The model under review builds one solid part; all positions refer to its coordinate system, in mm. Face numbers are marked on the shaded views. A direction names the side the tool comes from. Give positions to 0.01 mm unless a question says otherwise; leave off trailing zeros. Return JSON: item names as keys, results as strings. Group by question number.
from build123d import *

# Parameters (mm, degrees)
SKETCH1_W           = 30
SKETCH1_H           = 12
BOSS_EXTRUDE1_DEPTH = 5
CUT_EXTRUDE1_DEPTH  = 34.823069051
LPATTERN1_COUNT     = 10
LPATTERN1_PITCH     = 3.141592654
TAP1_D              = 2.459
TAP1_DEPTH          = 6
TAP1_TIP            = 0.738758131
TAP3_D              = 2.459
TAP3_DEPTH          = 6
TAP3_TIP            = 0.738758131


with BuildPart() as part:
    # Sketch1 → Boss-Extrude1 (new, symmetric)
    with BuildSketch(Plane.XY):
        with Locations((15, 6)):
            Rectangle(SKETCH1_W, SKETCH1_H)
    extrude(amount=BOSS_EXTRUDE1_DEPTH, both=True)

    # Sketch2 → Cut-Extrude1 (cut, through all)
    with BuildSketch(Plane.XY.offset(5)):
        with BuildLine():
            Line((-1.149368398, 12), (1.149368398, 12))
            Line((1.149368398, 12), (0.426229404, 10.013191943))
            ThreePointArc((0.426229404, 10.013191943), (0.27978293, 9.822339182), (0.050352355, 9.75))
            Line((0.050352355, 9.75), (-0.050352355, 9.75))
            ThreePointArc((-0.050352355, 9.75), (-0.27978293, 9.822339182), (-0.426229404, 10.013191943))
            Line((-0.426229404, 10.013191943), (-1.149368398, 12))
        make_face()
    cut_extrude1 = extrude(amount=-CUT_EXTRUDE1_DEPTH, mode=Mode.SUBTRACT)

    # LPattern1: Cut-Extrude1 ×10
    with Locations(*[(i * LPATTERN1_PITCH, 0, 0) for i in range(1, LPATTERN1_COUNT)]):
        add(cut_extrude1, mode=Mode.SUBTRACT)

    # Tap1
    with Locations(Plane(origin=(-45.41658703, 4.630780207, 5), x_dir=(-1, 0, 0), z_dir=(0, 0, 1))):
        with Locations((-55.41658703, -0.869219793)):
            Hole(TAP1_D / 2, depth=TAP1_DEPTH)
            with Locations((0, 0, -(TAP1_DEPTH + TAP1_TIP / 2))):  # 118° drill point
                Cone(0, TAP1_D / 2, TAP1_TIP, mode=Mode.SUBTRACT)

    # Tap3
    with Locations(Plane(origin=(-24.792169361, 5.708678804, 5), x_dir=(-1, 0, 0), z_dir=(0, 0, 1))):
        with Locations((-49.792169361, 0.208678804)):
            Hole(TAP3_D / 2, depth=TAP3_DEPTH)
            with Locations((0, 0, -(TAP3_DEPTH + TAP3_TIP / 2))):  # 118° drill point
                Cone(0, TAP3_D / 2, TAP3_TIP, mode=Mode.SUBTRACT)


solid = part.part
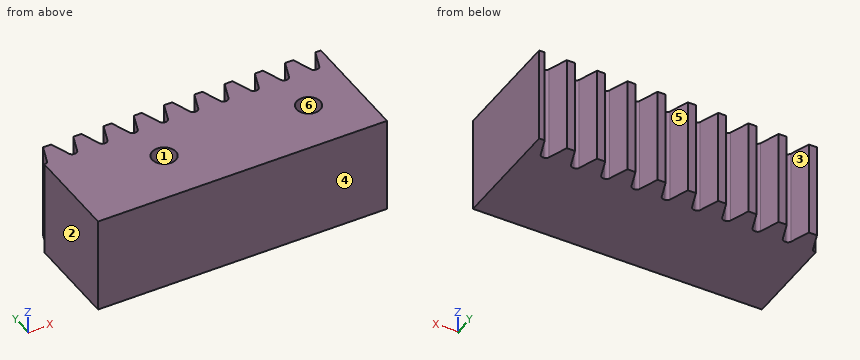
Item 1: Take a section at A-A (z = -0.25). State how many separate pieces and enclosed holes the cut face has, then the cut area to 3 significant figures.
Item 2: Mouldability with a two-part tool opening along Y and no side actions: class the marked faces 4, 5 and 6 as +Y half, -Y half, draft (parallel to the pull), parting line (faces both ways), or undercut.
Item 3: For L1, parallel to X at y = 5.5, z = 3.2; L2, parallel to Y at x = 12.25, z = -4.5; L3, parallel to Y at x = 25, z = 2.25, list the stretches that pass through material, from the lowest coordinate up. Write a range as from..to.
Item 4: Tool access review of the marked faces 1, 2 and 3: name each direction out of +Z, -Z, +X, -X, +Y, -Y from which nothing blocks a thin tool from reaching the whole face with its end or side.
Item 5: For P1, Ø2, axis at x = 25, y = 5.5, coming from the +Z side, flat-tipped, find the tip position at first contact; note if it passes through.
Check sheet entries:
{
 "1": {"separate pieces": "1", "enclosed holes": "2", "area": "319 mm^2"},
 "2": {"face 4": "-Y half", "face 5": "+Y half", "face 6": "undercut"},
 "3": {"L1": "x = 0..8.77, 11.23..23.77, 26.23..30", "L2": "y = 0..9.85", "L3": "y = 0..4.27, 6.73..9.76"},
 "4": {"face 1": "+Z", "face 2": "+Z, -Z, -X, +Y, -Y", "face 3": "+Z, -Z, +Y"},
 "5": {"P1": "stops at z = -1.14"}
}
